```python
from build123d import *

# Parameters (mm, degrees)
MAINBASESKETCH_W                       = 15.8
MAINBASESKETCH_H                       = 3.2
MAINBASEEXTRUDE_DEPTH                  = 7.9
STUDSSKETCH_R                          = 2.4
STUDSEXTRUDE_DEPTH                     = 1.6
STUDSPATTERN_COUNT                     = 2
STUDSPATTERN_PITCH                     = 8
STUDSPATTERN_COUNT_DIR2                = 2
STUDSPATTERN_PITCH_DIR2                = 8
MAINBASESHELL_T                        = -1.2
LCUTBLUE_DEPTH                         = 19.555463972
LCUTBLUE_DEPTH_BACK                    = 19.555463972
CUTADDEDTOLCUT_DEPTH                   = 2
MADESLIMCUTSKETCH_W                    = 7.9
MADESLIMCUTSKETCH_H                    = 7.9
MADESLIMCUT_DEPTH                      = 19.897228453
MADESLIMFILLEXT_REACH                  = 20.897
SKETCH33_W                             = 5.500952983
SKETCH33_H                             = 1.199047018
SLIMHOLEEXT_START                      = -0.2
SLIMHOLESKETCH_R                       = 1.25
SLIMHOLESKETCH_R_2                     = 0.75
SLIMHOLEEXT_DEPTH                      = 2
ANGLEDSLIMBASESWEEP_START              = 0.681967213
ANGLEDSLIMBASESWEEP_OUTLINE_W          = 7.9
ANGLEDSLIMBASESWEEP_OUTLINE_H          = 1.583745828
ANGLEDSLIMBASESWEEP_DEPTH              = 15.8
SHORTLEXTENDEDCUT_START                = -2
SHORTLEXTENDEDCUTSKETCH_W              = 13.4
SHORTLEXTENDEDCUTSKETCH_H              = 1.582792846
SHORTLEXTENDEDCUT_DEPTH                = 2
SHORTLUNDERSTUMPS_START                = -0.2
SHORTLUNDERSTUMPSKETCH_W               = 0.996828098
SHORTLUNDERSTUMPSKETCH_H               = 1.1
SHORTLUNDERSTUMPS_DEPTH                = 1.5
SHORTLUPPERCIRCLES_START               = -0.2
SHORTLUPPERCIRCLESSKETCH_R             = 2.45
SHORTLUPPERCIRCLESSKETCH_R_2           = 2
SHORTLUPPERCIRCLES_DEPTH               = 2
HOLESBASEHOLESHORT_START               = 0.681967213
HOLESBASEHOLESHORT_OUTLINE_W           = 7.48
HOLESBASEHOLESHORT_OUTLINE_H           = 1.583745828
HOLESBASEHOLESHORT_DEPTH               = 15.8
F_4UPPERCIRCLESTALLERLBASE_START       = -3.383745828
F_4UPPERCIRCLESTALLERLBASE_OUTLINE_R   = 2.45
F_4UPPERCIRCLESTALLERLBASE_OUTLINE_R_2 = 2
F_4UPPERCIRCLESTALLERLBASE_DEPTH       = 1.8
TALLERLBASEOUTERCHAMFER_R              = 1


# Read off the part's stored shape, not the designer's step: AngledSlimBaseSweep, HolesBaseHoleShort, 4UpperCirclesTallerLBase
with BuildPart() as part:
    # MainBaseSketch → MainBaseExtrude (new, symmetric)
    with BuildSketch(Plane.XY):
        with Locations((8.581967213, 1.6)):
            Rectangle(MAINBASESKETCH_W, MAINBASESKETCH_H)
    extrude(amount=MAINBASEEXTRUDE_DEPTH, both=True)

    # StudsSketch → StudsExtrude (add)
    with BuildSketch(Plane(origin=(0, 3.2, 0), x_dir=(1, 0, 0), z_dir=(0, 1, 0))):
        with Locations((4.581967213, 4)):
            Circle(STUDSSKETCH_R)
    studsextrude = extrude(amount=STUDSEXTRUDE_DEPTH)

    # StudsPattern: StudsExtrude 2 × 2
    with Locations(*[(j * STUDSPATTERN_PITCH_DIR2, 0, i * STUDSPATTERN_PITCH) for i in range(STUDSPATTERN_COUNT) for j in range(STUDSPATTERN_COUNT_DIR2) if (i, j) != (0, 0)]):
        add(studsextrude)

    # MainBaseShell
    mainbaseshell_openings = [part.faces().sort_by_distance(p)[0] for p in [
        (8.581967213, 0, 0),
    ]]
    offset(amount=MAINBASESHELL_T, openings=mainbaseshell_openings, kind=Kind.INTERSECTION)

    # LCUTBlueSketch → LCutBlue (cut, two sides: drawn at the far end of the back side and taken through both)
    with BuildSketch(Plane(origin=(0, 3.2, 0), x_dir=(1, 0, 0), z_dir=(0, 1, 0)).offset(-LCUTBLUE_DEPTH_BACK)):
        Polygon((8.581967213, 53.229874044), (8.581967213, 7.9), (8.581967213, 0), (16.481967213, 0), (61.811841258, 0), (125.917963912, 64.106122654), (72.688089868, 117.335996699), align=None)
    extrude(amount=LCUTBLUE_DEPTH + LCUTBLUE_DEPTH_BACK, mode=Mode.SUBTRACT)

    # CutAddedtoLSketch → CutAddedToLCut (add)
    with BuildSketch(Plane.XZ):
        Polygon((7.382920196, -6.7), (8.581967213, -6.7), (8.581967213, 0), (15.281967213, 0), (15.281967213, 1.199047018), (7.382920196, 1.199047018), (7.382920196, 0), align=None)
    extrude(amount=-CUTADDEDTOLCUT_DEPTH)

    # MadeSlimCutSketch → MadeSlimCut (cut, through all)
    with BuildSketch(Plane.XZ):
        with Locations((4.631967213, -3.95)):
            Rectangle(MADESLIMCUTSKETCH_W, MADESLIMCUTSKETCH_H)
    extrude(amount=-MADESLIMCUT_DEPTH, mode=Mode.SUBTRACT)

    # Sketch33 → MadeSlimFillExt (add, up to next)
    with BuildSketch(Plane.XZ, mode=Mode.PRIVATE) as madeslimfillext_sk1:
        with Locations((4.632443704, 0.599523509)):
            Rectangle(SKETCH33_W, SKETCH33_H)
    madeslimfillext_tool1 = extrude(madeslimfillext_sk1.sketch, amount=-MADESLIMFILLEXT_REACH, mode=Mode.PRIVATE) - part.part
    add(madeslimfillext_tool1.solids().sort_by_distance((4.632444, 0, 0.599524))[0])

    # SlimHoleSketch → SlimHoleExt (add)
    with BuildSketch(Plane.XZ.offset(-2).offset(SLIMHOLEEXT_START)):
        with Locations((8.581967213, 4)):
            Circle(SLIMHOLESKETCH_R)
        with Locations((8.581967213, 4)):
            Circle(SLIMHOLESKETCH_R_2, mode=Mode.SUBTRACT)
    extrude(amount=SLIMHOLEEXT_DEPTH)

    # AngledSlimBaseSweep outline → AngledSlimBaseSweep (add)
    with BuildSketch(Plane.YZ.offset(ANGLEDSLIMBASESWEEP_START)):
        with Locations((3.95, -0.791872914)):
            Rectangle(ANGLEDSLIMBASESWEEP_OUTLINE_W, ANGLEDSLIMBASESWEEP_OUTLINE_H)
    extrude(amount=ANGLEDSLIMBASESWEEP_DEPTH)

    # ShortLExtendedCutSketch → ShortLExtendedCut (cut)
    with BuildSketch(Plane.XZ.offset(SHORTLEXTENDEDCUT_START)):
        with Locations((8.581967213, 0.407650595)):
            Rectangle(SHORTLEXTENDEDCUTSKETCH_W, SHORTLEXTENDEDCUTSKETCH_H)
    extrude(amount=SHORTLEXTENDEDCUT_DEPTH, mode=Mode.SUBTRACT)

    # ShortLUnderStumpSketch → ShortLUnderStumps (add)
    with BuildSketch(Plane.XZ.offset(-2).offset(SHORTLUNDERSTUMPS_START)):
        with Locations((4.581764801, 0.166254172)):
            Rectangle(SHORTLUNDERSTUMPSKETCH_W, SHORTLUNDERSTUMPSKETCH_H)
        with Locations((8.57767054, 0.166254172)):
            Rectangle(SHORTLUNDERSTUMPSKETCH_W, SHORTLUNDERSTUMPSKETCH_H)
        with Locations((12.582169625, 0.166254172)):
            Rectangle(SHORTLUNDERSTUMPSKETCH_W, SHORTLUNDERSTUMPSKETCH_H)
    extrude(amount=SHORTLUNDERSTUMPS_DEPTH)

    # ShortLUpperCirclesSketch → ShortLUpperCircles (add)
    # profile 1 of 2: a face of its own
    with BuildSketch(Plane(origin=(0, 0, -1.583745828), x_dir=(-1, 0, 0), z_dir=(0, 0, -1)).offset(SHORTLUPPERCIRCLES_START)):
        with Locations(Location((-12.581967213, 3.95, 0), (0, 0, 90))):
            Circle(SHORTLUPPERCIRCLESSKETCH_R)
        with Locations(Location((-12.581967213, 3.95, 0), (0, 0, 90))):
            Circle(SHORTLUPPERCIRCLESSKETCH_R_2, mode=Mode.SUBTRACT)
    # profile 2 of 2: a face of its own
    with BuildSketch(Plane(origin=(0, 0, -1.583745828), x_dir=(-1, 0, 0), z_dir=(0, 0, -1)).offset(SHORTLUPPERCIRCLES_START)):
        with Locations(Location((-4.581967213, 3.95, 0), (0, 0, 270))):
            Circle(SHORTLUPPERCIRCLESSKETCH_R)
        with Locations(Location((-4.581967213, 3.95, 0), (0, 0, 270))):
            Circle(SHORTLUPPERCIRCLESSKETCH_R_2, mode=Mode.SUBTRACT)
    extrude(amount=SHORTLUPPERCIRCLES_DEPTH)

    # HolesBaseHoleShort outline → HolesBaseHoleShort (add)
    with BuildSketch(Plane.YZ.offset(HOLESBASEHOLESHORT_START)):
        with Locations((11.64, -0.791872914)):
            Rectangle(HOLESBASEHOLESHORT_OUTLINE_W, HOLESBASEHOLESHORT_OUTLINE_H)
    extrude(amount=HOLESBASEHOLESHORT_DEPTH)

    # 4UpperCirclesTallerLBase outline → 4UpperCirclesTallerLBase (add)
    # profile 1 of 2: a face of its own
    with BuildSketch(Plane.XY.offset(F_4UPPERCIRCLESTALLERLBASE_START)):
        with Locations((4.581967213, 11.95)):
            Circle(F_4UPPERCIRCLESTALLERLBASE_OUTLINE_R)
        with Locations((4.581967213, 11.95)):
            Circle(F_4UPPERCIRCLESTALLERLBASE_OUTLINE_R_2, mode=Mode.SUBTRACT)
    # profile 2 of 2: a face of its own
    with BuildSketch(Plane.XY.offset(F_4UPPERCIRCLESTALLERLBASE_START)):
        with Locations((12.581967213, 11.95)):
            Circle(F_4UPPERCIRCLESTALLERLBASE_OUTLINE_R)
        with Locations((12.581967213, 11.95)):
            Circle(F_4UPPERCIRCLESTALLERLBASE_OUTLINE_R_2, mode=Mode.SUBTRACT)
    extrude(amount=F_4UPPERCIRCLESTALLERLBASE_DEPTH)

    # TallerLBaseOuterChamfer
    tallerlbaseouterchamfer_edges = [part.edges().sort_by_distance(p)[0] for p in [
        (16.481967213, 15.38, -0.791872914),
        (0.681967213, 15.38, -0.791872914),
    ]]
    fillet(tallerlbaseouterchamfer_edges, radius=TALLERLBASEOUTERCHAMFER_R)


solid = part.part
```
For this review, take the finished solid that the model builds, in its own axes (mm). A direction names the side the tool comes from. Coordinates: 2 decimals unless noted, no trailing zeros. Loops run counter-clockwise (first coordinate to the right, second up) from the corner with the lowest first, then second, coordinate; pieces in that order, holes last. Notation, with made-up numbers: (65, -2.5) - (88, -2.5) arc R14 ccw to (88, 16.5) - close; hole circle Ø7 at (65.5, 42.5). An arc over 180 degrees is marked (long way). Use one line per item in the form item = value. Start each with the question number.
1) For pin 1 (5 mm diameter, centred on y = 11, z = 1.5, fed in from +X); pin 2 (2 mm diameter, centred on x = 10, z = 2.5, fed in from -Y); pin 3 (1.2 mm diameter, centred on x = 8.58, z = 4, fed in from -Y); pin 4 (1.2 mm diameter, centred on x = 5, y = 4.5, fed in from -Z), all flat-tipped, find the tip position at first contact; note any pin that passes through.
2) Draft analysis for pull direction X (two halves, no side actions). For faces 4 (the face through (16.482, 3, 2)), 5 (the face through (5.08, 1, 0)), 6 (the face through (8, 2, 7.9)), state which applies: released by +X, released by -X, zero draft, split by the parting line, or undercut.
3) Take a section at C-C (y = 11.95). State the section outline as (x, z) points.
4) To check wall thickness, follow probe 1 along X at (y, z) = (3.95, -2.2); probe 2 along Y at (x, z) = (11.25, 6.5); probe 3 along Y at (x, z) = (12, 1.75). State the ranges of each line that lie inside material, in increasing order. Write a range as from..to.
5) For faces 1 (the face through (4.26, 14.38, -2.5)), 2 (the face through (8, 3.2, 4)), 3 (the face through (8.6, 0.7, 0.2)), list the 3-axis set-ups (+Z, -Z, +X, -X, +Y, -Y) from which the entire face can be reached by the end or side of a thin tool; tool diameter is ignored.
6) Take a section at A-A (y = 3.95). State the section outline as (x, z) points, plus the area to 3 significant figures.
From the geometry:
q1.pin_1 = 16.48
q1.pin_2 = 0.2
q1.pin_3 = 2
q1.pin_4 = -1.58
q2.face_4 = released by +X
q2.face_5 = undercut
q2.face_6 = zero draft
q3.outline = (0.68, -1.58) - (2.13, -1.58) - (2.13, -3.38) - (2.58, -3.38) - (2.58, -1.58) - (6.58, -1.58) - (6.58, -3.38) - (7.03, -3.38) - (7.03, -1.58) - (10.13, -1.58) - (10.13, -3.38) - (10.58, -3.38) - (10.58, -1.58) - (14.58, -1.58) - (14.58, -3.38) - (15.03, -3.38) - (15.03, -1.58) - (16.48, -1.58) - (16.48, 0) - (0.68, 0) - close
q4.probe_1 = 2.13..2.58, 6.58..7.03, 10.13..10.58, 14.58..15.03
q4.probe_2 = 2..3.2
q4.probe_3 = 2..4.8
q5.face_1 = -Z
q5.face_2 = +Y
q5.face_3 = -Y
q6.outline = (0.68, -1.58) - (2.13, -1.58) - (2.13, -3.38) - (2.58, -3.38) - (2.58, -1.58) - (6.58, -1.58) - (6.58, -3.38) - (7.03, -3.38) - (7.03, -1.58) - (10.13, -1.58) - (10.13, -3.38) - (10.58, -3.38) - (10.58, -1.58) - (14.58, -1.58) - (14.58, -3.38) - (15.03, -3.38) - (15.03, -1.58) - (16.48, -1.58) - (16.48, 0) - (0.68, 0) - close; circle Ø4.8 at (4.58, 4); circle Ø4.8 at (12.58, 4)
q6.area = 64.5 mm2
